Check sheet for the modelled part. Datum: model origin and axes. Units: mm. Give positions to 0.01 mm unless a question says otherwise; leave off trailing zeros. Order: outer loops, then holes, each group sorted by start corner. A loop starts at its lowest first (then second) coordinate and runs counter-clockwise, first axis right, second up.
```python
from build123d import *

# Parameters (mm, degrees)
BOSS_EXTRUDE1_DEPTH = 6.35
CUT_EXTRUDE1_REACH  = 8.35
SKETCH2_R           = 1.0795


with BuildPart() as part:
    # Sketch1 → Boss-Extrude1 (new body)
    with BuildSketch(Plane(origin=(0, 0, 0), x_dir=(0, 1, 0), z_dir=(0, 0, 1))):
        with BuildLine():
            Line((-9.525, 16.497783942), (-6.35, 10.998522628))
            ThreePointArc((-6.35, 10.998522628), (0, 12.7), (6.35, 10.998522628))
            Line((6.35, 10.998522628), (9.525, 16.497783942))
            ThreePointArc((9.525, 16.497783942), (0, 19.05), (-9.525, 16.497783942))
        make_face()
    extrude(amount=BOSS_EXTRUDE1_DEPTH)

    # Sketch2 → Cut-Extrude1 (cut, up to next)
    with BuildSketch(Plane.XY.offset(6.35), mode=Mode.PRIVATE) as cut_extrude1_sk1:
        with Locations((-15.057884182, 5.027499276)):
            Circle(SKETCH2_R)
    cut_extrude1_tool1 = extrude(cut_extrude1_sk1.sketch, amount=-CUT_EXTRUDE1_REACH, mode=Mode.PRIVATE) & part.part
    add(cut_extrude1_tool1.solids().sort_by_distance((-15.057884, 5.027499, 6.35))[0], mode=Mode.SUBTRACT)
    # Sketch2 → Cut-Extrude1 (cut, up to next)
    with BuildSketch(Plane.XY.offset(6.35), mode=Mode.PRIVATE) as cut_extrude1_sk2:
        with Locations((-15.057884182, -5.027499276)):
            Circle(SKETCH2_R)
    cut_extrude1_tool2 = extrude(cut_extrude1_sk2.sketch, amount=-CUT_EXTRUDE1_REACH, mode=Mode.PRIVATE) & part.part
    add(cut_extrude1_tool2.solids().sort_by_distance((-15.057884, -5.027499, 6.35))[0], mode=Mode.SUBTRACT)


solid = part.part
```
(1) Cross-section at C-C on y = 7.75. Enter the section's corners in (x, z), then the cut area to 3 significant figures.
Response values:
outline: (-17.4, 0) - (-13.42, 0) - (-13.42, 6.35) - (-17.4, 6.35) - close
area: 25.3 mm2
(2) Release check for a two-part mould opening along X. For faces 1 (the face through (-13.79, -7.96, 3.13)), 2 (the face through (-14.061, 4.614, 3.219)), 3 (the face through (-15, 0, 6.35)), 4 (the face through (-19.05, 0.14, 3.13)) record: released by +X, released by -X, zero draft, split by the parting line, or undercut.
Response values:
face 1: released by +X
face 2: undercut
face 3: zero draft
face 4: released by -X
(3) Cross-section at B-B on z = 2. Count the separate pieces of the cut face and the enclosed holes in it, then the cut area to 3 significant figures.
Response values:
separate pieces: 1
enclosed holes: 2
area: 98.2 mm2
(4) Cross-section at A-A on x = -14.5. Enter the section's corners in (y, z), then the cut area to 3 significant figures.
Response values:
outline: (-8.37, 0) - (-5.95, 0) - (-5.95, 6.35) - (-8.37, 6.35) - close; (-4.1, 0) - (4.1, 0) - (4.1, 6.35) - (-4.1, 6.35) - close; (5.95, 0) - (8.37, 0) - (8.37, 6.35) - (5.95, 6.35) - close
area: 82.8 mm2
(5) Material ranges on L1, parallel to Y at x = -15.5, z = 1.5; L2, parallel to Y at x = -14.25, z = 4.75; L3, parallel to X at y = -5.5, z = 1.75, recorded low to high.
Response values:
L1: y = -8.95 to -6.01, -4.04 to 4.04, 6.01 to 8.95
L2: y = -8.23 to -5.74, -4.31 to 4.31, 5.74 to 8.23
L3: x = -18.24 to -16.03, -14.09 to -11.45
(6) Cross-section at D-D on x = -13. Enter the section's corners in (y, z), then the cut area to 3 significant figures.
Response values:
outline: (-7.51, 0) - (7.51, 0) - (7.51, 6.35) - (-7.51, 6.35) - close
area: 95.3 mm2
